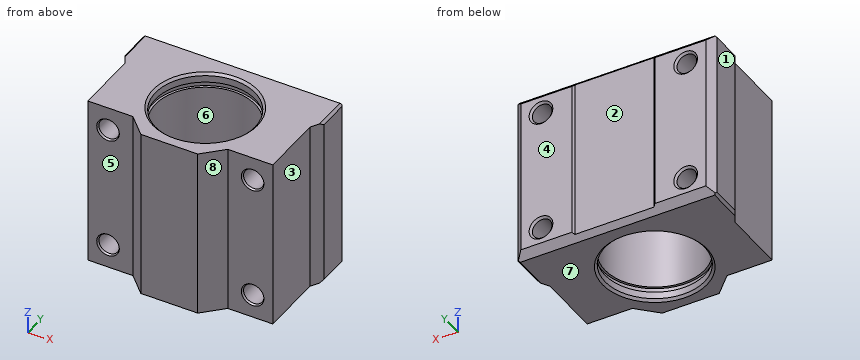
```python
from build123d import *

# Parameters (mm, degrees)
BOSS_EXTRUDE1_DEPTH     = 36
CUT_EXTRUDE1_DEPTH      = 21
CUT_EXTRUDE1_DEPTH_BACK = 21
SKETCH2_W               = 54
SKETCH2_H               = 56
CUT_EXTRUDE2_DEPTH      = 28
CUT_EXTRUDE2_DEPTH_BACK = 28
SKETCH4_W               = 52
SKETCH4_H               = 46


with BuildPart() as part:
    # Sketch1 → Boss-Extrude1 (new body)
    with BuildSketch(Plane.XY):
        Polygon((-21, 13.5), (-21, 7), (-19.5, 4.401923789), (-19.5, -9), (-10, -9), (-6, -13), (6, -13), (10, -9), (19.5, -9), (19.5, 4.401923789), (21, 7), (21, 13.5), (19.5, 15), (8.75, 15), (8.35, 14.6), (-8.35, 14.6), (-8.75, 15), (-19.5, 15), align=None)
    extrude(amount=BOSS_EXTRUDE1_DEPTH)

    # Sketch2 → Cut-Extrude1 (cut, two sides: drawn at the far end of the back side and taken through both)
    with BuildSketch(Plane(origin=(0, 0, 0), x_dir=(0, 0, -1), z_dir=(1, 0, 0)).offset(-CUT_EXTRUDE1_DEPTH_BACK)):
        with Locations((-18, 0)):
            Rectangle(SKETCH2_W, SKETCH2_H)
        Polygon((-36, 13.5), (-36, -13), (0, -13), (0, 13.5), (-1.5, 15), (-34.5, 15), align=None, mode=Mode.SUBTRACT)
    extrude(amount=CUT_EXTRUDE1_DEPTH + CUT_EXTRUDE1_DEPTH_BACK, mode=Mode.SUBTRACT)

    # Sketch3 → Cut-Revolve1 (revolve, cut)
    with BuildSketch(Plane(origin=(0, 0, 0), x_dir=(0, 0, -1), z_dir=(1, 0, 0)), mode=Mode.PRIVATE) as cut_revolve1_sk:
        Polygon((-36, 0), (-36, 11), (-35.5, 10.5), (-34.04, 10.5), (-34.04, 11), (-32.89, 11), (-32.89, 10.5), (-3.11, 10.5), (-3.11, 11), (-1.96, 11), (-1.96, 10.5), (-0.5, 10.5), (0, 11), (0, 0), align=None)
    revolve(cut_revolve1_sk.sketch.rotate(Axis((0, 0, 0), (0, 0, 1)), 270), axis=Axis((0, 0, 0), (0, 0, 1)), mode=Mode.SUBTRACT)

    # Sketch4 → Cut-Extrude2 (cut, two sides: drawn at the far end of the back side and taken through both)
    with BuildSketch(Plane(origin=(0, 0, 0), x_dir=(1, 0, 0), z_dir=(0, 1, 0)).offset(-CUT_EXTRUDE2_DEPTH_BACK)):
        with Locations((0, -18)):
            Rectangle(SKETCH4_W, SKETCH4_H)
        Polygon((-21, -0.5), (-21, -35.5), (-20.5, -36), (20.5, -36), (21, -35.5), (21, -0.5), (20.5, 0), (-20.5, 0), align=None, mode=Mode.SUBTRACT)
    extrude(amount=CUT_EXTRUDE2_DEPTH + CUT_EXTRUDE2_DEPTH_BACK, mode=Mode.SUBTRACT)

    # Sketch5 → Cut-Revolve2 (revolve, cut)
    with BuildSketch(Plane(origin=(15.25, 0, 0), x_dir=(0, 0, -1), z_dir=(1, 0, 0)), mode=Mode.PRIVATE) as cut_revolve2_sk:
        Polygon((-5, 15), (-2.5, 15), (-2.933, 14.567), (-2.933, 1), (-2.85, 1), (-2.85, -8.6), (-2.619059892, -9), (-5, -9), align=None)
    revolve(cut_revolve2_sk.sketch.rotate(Axis((15.25, -9, 5), (0, 1, 0)), 180), axis=Axis((15.25, -9, 5), (0, 1, 0)), mode=Mode.SUBTRACT)

    # Sketch6 → Cut-Revolve3 (revolve, cut)
    with BuildSketch(Plane(origin=(15.25, 0, 0), x_dir=(0, 0, -1), z_dir=(1, 0, 0)), mode=Mode.PRIVATE) as cut_revolve3_sk:
        Polygon((-31, 15), (-28.5, 15), (-28.933, 14.567), (-28.933, 1), (-28.85, 1), (-28.85, -8.6), (-28.619059892, -9), (-31, -9), align=None)
    revolve(cut_revolve3_sk.sketch.rotate(Axis((15.25, -9, 31), (0, 1, 0)), 180), axis=Axis((15.25, -9, 31), (0, 1, 0)), mode=Mode.SUBTRACT)

    # Sketch7 → Cut-Revolve4 (revolve, cut)
    with BuildSketch(Plane(origin=(-15.25, 0, 0), x_dir=(0, 0, -1), z_dir=(1, 0, 0)), mode=Mode.PRIVATE) as cut_revolve4_sk:
        Polygon((-5, 15), (-2.5, 15), (-2.933, 14.567), (-2.933, 1), (-2.85, 1), (-2.85, -8.6), (-2.619059892, -9), (-5, -9), align=None)
    revolve(cut_revolve4_sk.sketch.rotate(Axis((-15.25, -9, 5), (0, 1, 0)), 180), axis=Axis((-15.25, -9, 5), (0, 1, 0)), mode=Mode.SUBTRACT)

    # Sketch8 → Cut-Revolve5 (revolve, cut)
    with BuildSketch(Plane(origin=(-15.25, 0, 0), x_dir=(0, 0, -1), z_dir=(1, 0, 0)), mode=Mode.PRIVATE) as cut_revolve5_sk:
        Polygon((-31, 15), (-28.5, 15), (-28.933, 14.567), (-28.933, 1), (-28.85, 1), (-28.85, -8.6), (-28.619059892, -9), (-31, -9), align=None)
    revolve(cut_revolve5_sk.sketch.rotate(Axis((-15.25, -9, 31), (0, 1, 0)), 180), axis=Axis((-15.25, -9, 31), (0, 1, 0)), mode=Mode.SUBTRACT)


solid = part.part
```
Geometry: final body of the model. Coordinates: model frame, mm. Face numbers are marked on the shaded views. A direction names the side the tool comes from. Round coordinates to 2 decimals unless told otherwise and drop trailing zeros. Use one line per item in the form item = value. Start each with the question number.
1) Access query for the marked faces 1, 2, 3, 4 and 5. Directions: +Z, -Z, +X, -X, +Y, -Y. A direction counts if a zero-diameter tool reaches every point of the face in a straight line with its end or side. Return the directions, or none.
2) Draft query along Y for the marked faces 6, 7 and 8. Return one class per face: released by +Y, released by -Y, zero draft, split by the parting line, or undercut.
3) Section A-A on y = 0. Give the number of separate pieces and of enclosed holes in the cut face, then the cut area to 3 significant figures.
4) Line query: L1, parallel to Y at x = 0, z = 21; L2, parallel to X at y = 8, z = 31; L3, parallel to Z at x = -14.5, y = 0.5. Output: solid intervals per line, ascending.
5) First-contact query: P1, Ø1.3, axis at x = -15.5, z = 5, coming from the -Y side; P2, Ø6.5, axis at x = -15.25, z = 5, coming from the -Y side; P3, Ø6.5, axis at y = -1.5, z = 25.5, coming from the -X side; P4, Ø5, axis at x = 7, z = 26.5, coming from the -Y side. Flat tips, straight axial feed; report the tip coordinate or a pass-through.
Response:
q1.face_1 = +Z, -Z, -X, +Y, -Y
q1.face_2 = +Z, -Z, +Y
q1.face_3 = +Z, -Z, +X, -Y
q1.face_4 = +Z, -Z, +X, -X, +Y
q1.face_5 = +Z, -Z, -X, -Y
q2.face_6 = undercut
q2.face_7 = zero draft
q2.face_8 = released by -Y
q3.separate_pieces = 2
q3.enclosed_holes = 4
q3.area = 587 mm^2
q4.L1 = -13 to -10.5, 10.5 to 14.6
q4.L2 = -21 to -17.32, -13.18 to -6.8, 6.8 to 13.18, 17.32 to 21
q4.L3 = 0 to 2.99, 7.01 to 28.99, 33.01 to 36
q5.P1 = through
q5.P2 = -9
q5.P3 = -19.5
q5.P4 = -13
